```python
from build123d import *

# Parameters (mm, degrees)
SKICA1_W                 = 40.8
SKICA1_H                 = 38
P_IDAT_VYSUNUT_M1_DEPTH  = 5
SKICA2_R                 = 1.2
ODEBRAT_VYSUNUT_M1_DEPTH = 51.8
ODEBRAT_VYSUNUT_M2_DEPTH = 51.8


with BuildPart() as part:
    # Skica1 → Přidat vysunutím1 (new body)
    with BuildSketch(Plane.XY):
        Polygon((0, 86), (0, 0), (50.8, 0), (50.8, 86), (45.8, 86), (45.8, 48), (5, 48), (5, 86), align=None)
        with Locations((25.4, 24)):
            Rectangle(SKICA1_W, SKICA1_H, mode=Mode.SUBTRACT)
    extrude(amount=P_IDAT_VYSUNUT_M1_DEPTH)

    # Skica2 → Odebrat vysunutím1 (cut, through all)
    with BuildSketch(Plane(origin=(50.8, 0, 0), x_dir=(0, 0, -1), z_dir=(1, 0, 0))):
        with BuildLine():
            Line((-5, 86), (-5, 83.5))
            ThreePointArc((-5, 83.5), (-4.267766969, 85.267766937), (-2.500000046, 86))
            Line((-2.500000046, 86), (-5, 86))
        make_face()
        with BuildLine():
            Line((0, 86), (-2.500000046, 86))
            ThreePointArc((-2.500000046, 86), (-0.732233063, 85.267766969), (0, 83.5))
            Line((0, 83.5), (0, 86))
        make_face()
        with Locations((-2.5, 83.5)):
            Circle(SKICA2_R)
    extrude(amount=-ODEBRAT_VYSUNUT_M1_DEPTH, mode=Mode.SUBTRACT)

    # Skica3 → Odebrat vysunutím2 (cut, through all)
    with BuildSketch(Plane(origin=(50.8, 0, 0), x_dir=(0, 0, -1), z_dir=(1, 0, 0))):
        with BuildLine():
            ThreePointArc((-2.5, 0), (-4.267766953, 0.732233047), (-5, 2.5))
            Line((-5, 2.5), (-5, 0))
            Line((-5, 0), (-2.5, 0))
        make_face()
        with BuildLine():
            ThreePointArc((0, 2.5), (-0.732233047, 0.732233047), (-2.5, 0))
            Line((-2.5, 0), (0, 0))
            Line((0, 0), (0, 2.5))
        make_face()
    extrude(amount=-ODEBRAT_VYSUNUT_M2_DEPTH, mode=Mode.SUBTRACT)


solid = part.part
```
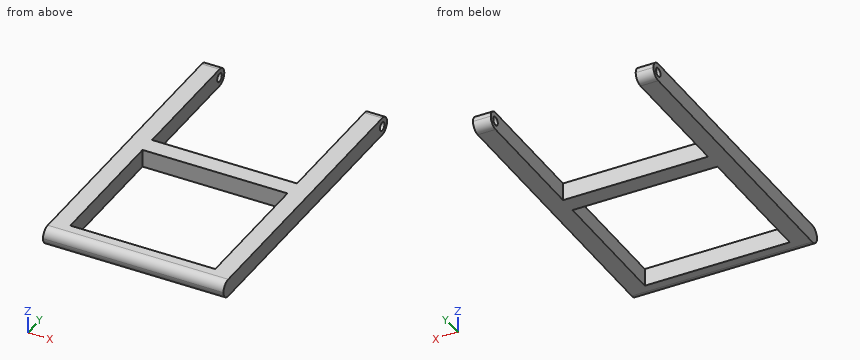
Part model, mm, in its own coordinate system. Round coordinates to 2 decimals unless told otherwise and drop trailing zeros. Order: outer loops, then holes, each group sorted by start corner. A loop starts at its lowest first (then second) coordinate and runs counter-clockwise, first axis right, second up. Notation, with made-up numbers: M -15.75,-36 L -9.75,-36 A16 ccw -9.75,-10 Z; hole C 73.5,26.5 d6. An arc over 180 degrees is marked long. Answer in a Markdown table with one row per item. Add a question column.
Q1. Cut at A-A on y = 23. Give the cut face in (x, z), and give its area (3 significant figures).
Q2. Pin check, flat tip, straight feed: pin 1 (1 mm diameter, centred on x = 11.5, z = 3.5, fed in from +Y). Stop position of the tip, or through.
Q3. Wall check: L1, parallel to X at y = 80.5, z = 2.85; L2, parallel to Z at x = 47.4, y = 83.5; L3, parallel to Y at x = 41.5, z = 2.5. Give the ranges that are in metal, low to high. Write a range as from..to.
Q4. Cut at B-B on x = 42.5. Give the cut face in (y, z).
Established:
| question | item | result |
|---|---|---|
| 1 | outline | M 0,0 L 5,0 L 5,5 L 0,5 Z; M 45.8,0 L 50.8,0 L 50.8,5 L 45.8,5 Z |
| 1 | area | 50.0 mm2 |
| 2 | pin 1 | stops at y = 48 |
| 3 | L1 | x = 0..5, 45.8..50.8 |
| 3 | L2 | z = 0..1.3, 3.7..5 |
| 3 | L3 | y = 0..5, 43..48 |
| 4 | outline | M 2.5,0 L 5,0 L 5,5 L 2.5,5 A2.5 ccw Z; M 43,0 L 48,0 L 48,5 L 43,5 Z |
